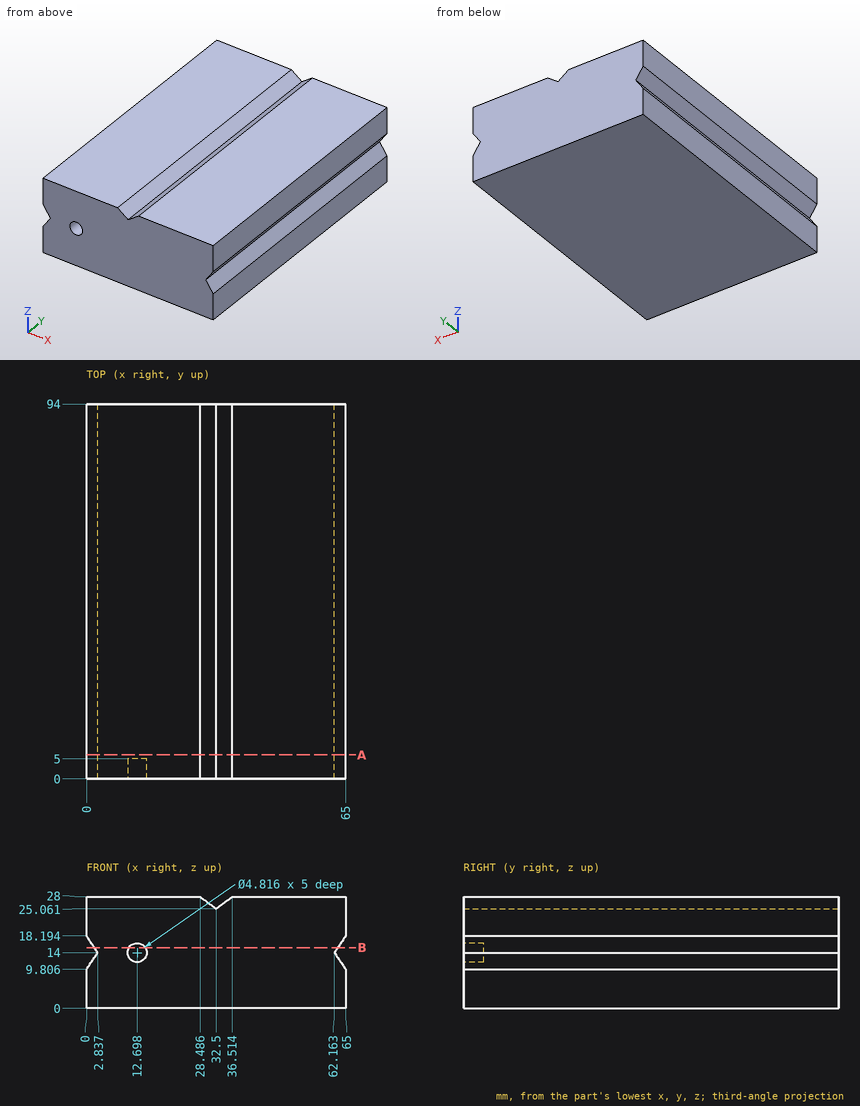
For this review, use the dimensioned drawing (mm, ordinates from the lowest corner) and the shaded views. Round coordinates to 2 decimals unless told otherwise and drop trailing zeros. Write each loop counter-clockwise with the first axis right and the second up, starting at its lowest first coordinate (ties: lowest second). Pieces come first, ordered by that corner, then holes. Notation, with made-up numbers: (65.5, -38) -> (120.5, -38) arc R18 ccw to (120.5, -7) -> close; hole circle Ø1 at (54, 85.25). An arc over 180 degrees is marked (long way). Answer in a Markdown table with one row per item.
Q1. To check wall thickness, follow L1, parallel to X at y = 2.6, z = 14 (1 decimal); L2, parallel to Z at x = 36.5, y = 13.5; L3, parallel to X at y = 77.5, z = 26.75 (1 decimal). State the ranges of each line that lie inside material, in increasing order. Write a range as [from, to].
The answers:
| item | result |
|---|---|
| L1 | [2.8, 10.3], [15.1, 62.2] |
| L2 | [0, 27.99] |
| L3 | [0, 30.2], [34.8, 65] |
Q2. Take a section at A-A, the plane y = 6. State the section outline as (x, z) points (1 decimal), then the cut area to 3 significant figures.
The answers:
| item | result |
|---|---|
| outline | (0, 0) -> (65, 0) -> (65, 9.8) -> (62.2, 14) -> (65, 18.2) -> (65, 28) -> (36.5, 28) -> (32.5, 25.1) -> (28.5, 28) -> (0, 28) -> (0, 18.2) -> (2.8, 14) -> (0, 9.8) -> close |
| area | 1,780 mm² |
Q3. Clearance check with a flat-ended pin moving along its axis: pin 1 Ø1 at (y, z) = (17, 17.5) entering from -X. State where the tip first meets the part, or that it passes through.
The answers:
| item | result |
|---|---|
| pin 1 | x = 0.13 |
Q4. Take a section at B-B, the plane z = 15.25. State the section outline as (x, y) points (1 decimal).
The answers:
| item | result |
|---|---|
| outline | (2, 0) -> (10.6, 0) -> (10.6, 5) -> (14.8, 5) -> (14.8, 0) -> (63, 0) -> (63, 94) -> (2, 94) -> close |
